Geometry: see drawing. Coordinates: mm, zero at the bounding-box minimum. A direction names the side the tool comes from. Coordinates: 2 decimals unless noted, no trailing zeros. Write each loop counter-clockwise with the first axis right and the second up, starting at its lowest first coordinate (ties: lowest second). Pieces come first, ordered by that corner, then holes.
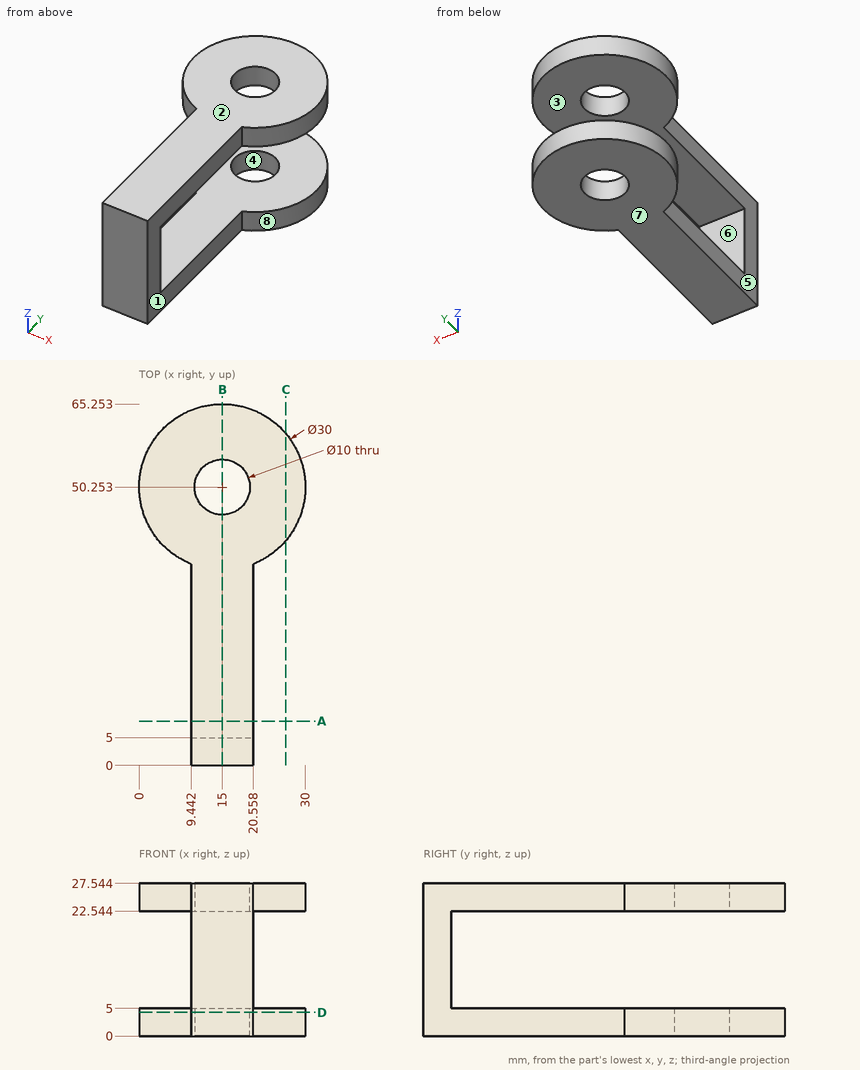
Item 1: Section D-D, the plane z = 4.25. Output: boundary loops of the cut face in (x, y), plus the area to 3 significant figures.
Derived:
outline: (9.44, 0) - (20.56, 0) - (20.56, 36.32) arc R15 ccw (long way) to (9.44, 36.32) - close; hole circle Ø10 at (15, 50.25)
area: 1,020 mm2
Item 2: Section A-A, the plane y = 8. Output: boundary loops of the cut face in (x, z), plus the area to 3 significant figures.
Derived:
outline: (9.44, 0) - (20.56, 0) - (20.56, 5) - (9.44, 5) - close; (9.44, 22.54) - (20.56, 22.54) - (20.56, 27.54) - (9.44, 27.54) - close
area: 111 mm2
Item 3: Pull-direction query (Z, two-part tool) for the marked faces 6, 7 and 8; classes: released by +Z, released by -Z, zero draft, split by the parting line, or undercut.
Derived:
face 6: undercut
face 7: released by -Z
face 8: zero draft
Item 4: Set-up query: the marked faces 1, 2, 3, 4 and 5. Return all of +Z, -Z, +X, -X, +Y, -Y with unobstructed straight access to the full face (end or side cutting, diameter ignored); none if empty.
Derived:
face 1: +Z, -Z, +X, -Y
face 2: +Z, +X, -X, +Y, -Y
face 3: +X, -X, +Y
face 4: +Z, -Z
face 5: +Z, -Z, -X, -Y
Item 5: Pin query (flat end, axial travel): pin 1 (12 mm diameter, centred on y = 50, z = 14, fed in from -X); pin 2 (9 mm diameter, centred on x = 15, z = 18, fed in from +Y); pin 3 (1 mm diameter, centred on y = 55, z = 23, fed in from -X); pin 4 (14 mm diameter, centred on y = 20.5, z = 17, fed in from -X). Return the tip coordinate at first contact, or that it passes through.
Derived:
pin 1: passes through
pin 2: stops at y = 5
pin 3: stops at x = 0.61
pin 4: stops at x = 9.44
Item 6: Section C-C, the plane x = 26.5. Output: boundary loops of the cut face in (y, z), plus the area to 3 significant figures.
Derived:
outline: (40.62, 0) - (59.88, 0) - (59.88, 5) - (40.62, 5) - close; (40.62, 22.54) - (59.88, 22.54) - (59.88, 27.54) - (40.62, 27.54) - close
area: 193 mm2
Item 7: Section B-B, the plane x = 15. Output: boundary loops of the cut face in (y, z).
Derived:
outline: (0, 0) - (45.25, 0) - (45.25, 5) - (5, 5) - (5, 22.54) - (45.25, 22.54) - (45.25, 27.54) - (0, 27.54) - close; (55.25, 0) - (65.25, 0) - (65.25, 5) - (55.25, 5) - close; (55.25, 22.54) - (65.25, 22.54) - (65.25, 27.54) - (55.25, 27.54) - close
Item 8: Material intervals for probe 1 along Y at (x, z) = (15, 25.85); probe 2 along Z at (x, y) = (22.5, 47); probe 3 along Y at (x, z) = (18, 20.25), sorted ascending.
Derived:
probe 1: y = 0 to 45.25, 55.25 to 65.25
probe 2: z = 0 to 5, 22.54 to 27.54
probe 3: y = 0 to 5
